For this review, use the dimensioned drawing (mm, ordinates from the lowest corner) and the shaded views. Round coordinates to 2 decimals unless told otherwise and drop trailing zeros. Order: outer loops, then holes, each group sorted by start corner. A loop starts at its lowest first (then second) coordinate and runs counter-clockwise, first axis right, second up. Notation, with made-up numbers: (66, 61.5) - (97, 61.5) arc R24 cw to (97, 72.5) - close; hole circle Ø1 at (13.25, -28). An arc over 180 degrees is marked (long way). Write item = value, one per line.
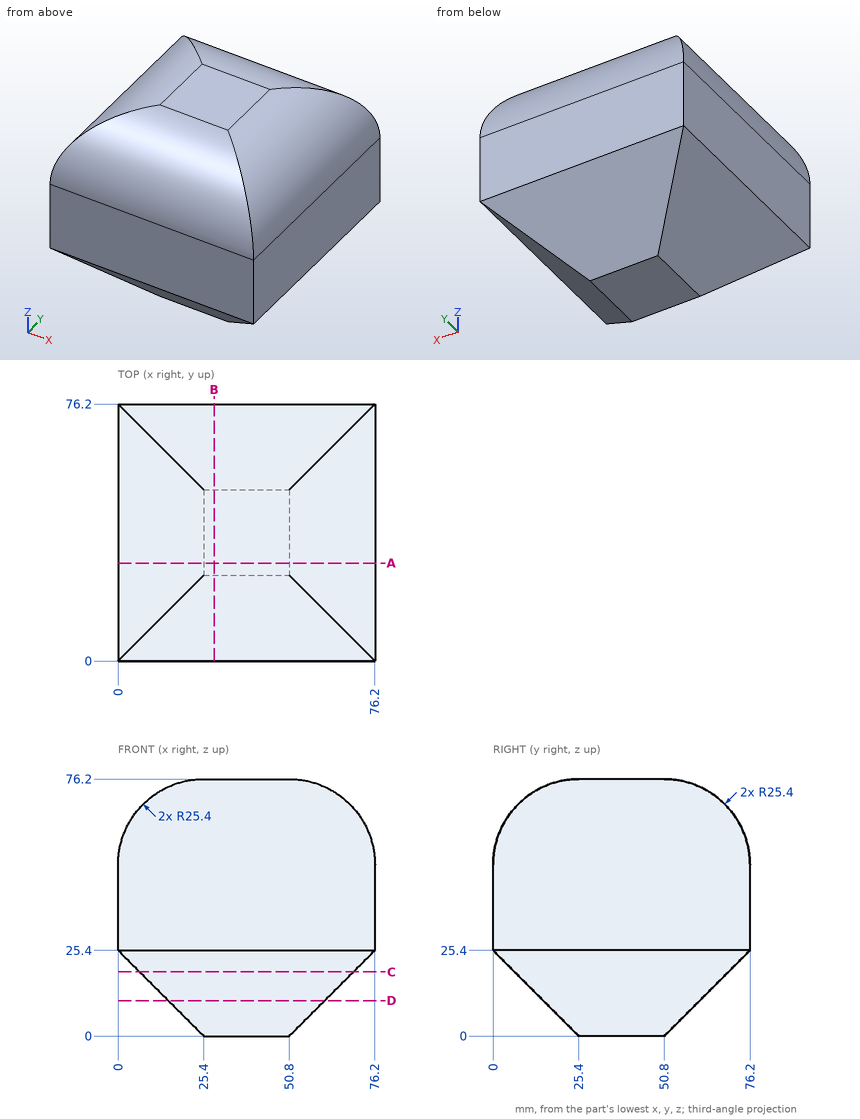
Item 1: Take a section at D-D, the plane z = 10.5. State the section outline as (x, y) points, and give its area (3 significant figures).
Data:
outline = (14.9, 14.9) - (61.3, 14.9) - (61.3, 61.3) - (14.9, 61.3) - close
area = 2,150 mm2
Item 2: Take a section at A-A, the plane y = 29. State the section outline as (x, z) points.
Data:
outline = (0, 25.4) - (25.4, 0) - (50.8, 0) - (76.2, 25.4) - (76.2, 50.8) arc R25.4 ccw to (50.8, 76.2) - (25.4, 76.2) arc R25.4 ccw to (0, 50.8) - close
Item 3: Insertion check: P1, Ø10, axis at y = 27, z = 65.5, coming from the +X side; P2, Ø6, axis at x = 68.5, y = 63, coming from the +Z side; P3, Ø6, axis at y = 20, z = 18.5, coming from the +X side. Each pin has a flat end and moves straight along its axis. Give the tip position at first contact, or say it passes through.
Data:
P1 = 74.27
P2 = 71.51
P3 = 72.3
Item 4: For line 1 along X through (y, z) = (33, 20); line 2 along Y through (x, z) = (15, 73); line 3 along X through (y, z) = (28.5, 7.5), list the stretches that pass through material, from the lowest coordinate up. Write a range as [from, to].
Data:
line_1 = [5.4, 70.8]
line_2 = [13.06, 63.14]
line_3 = [17.9, 58.3]
Item 5: Take a section at C-C, the plane z = 19. State the section outline as (x, y) points.
Data:
outline = (6.4, 6.4) - (69.8, 6.4) - (69.8, 69.8) - (6.4, 69.8) - close
